The figure shows three views and two pictorial views of one solid part (mm, origin at its lowest corner). Answer the questions. Give positions to 0.01 mm unless a question says otherwise; leave off trailing zeros. Write each loop counter-clockwise with the first axis right and the second up, starting at its lowest first coordinate (ties: lowest second). Pieces come first, ordered by that corner, then holes. Notation, with made-up numbers: M 48,68 L 86,68 A28 ccw 86,107 Z; hole C 30.25,8 d10. An arc over 180 degrees is marked long. Return JSON: item names as keys, results as strings.
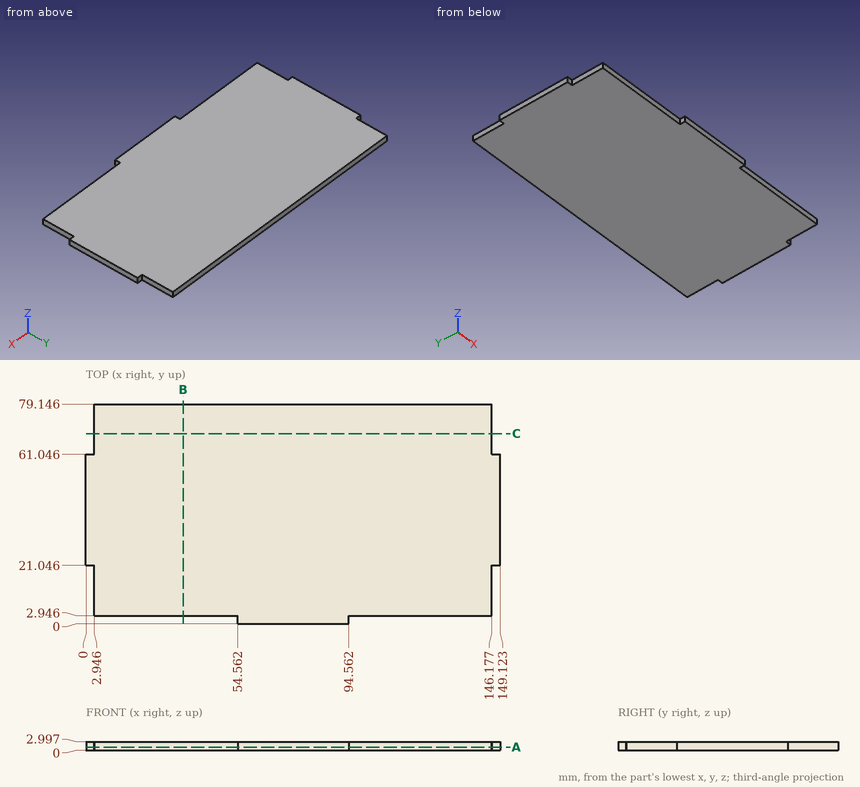
Item 1: Find the intervals of material crossed by line 1 (X direction, y = 64, z = 0.45); line 2 (Y direction, x = 96, z = 0.2), in increasing order.
Geometry results:
{"line 1": "x = 2.95 to 146.18", "line 2": "y = 2.95 to 79.15"}
Item 2: A cutting plane is placed at A-A, the plane z = 1.1. Write down the section's boundary in (x, y).
Geometry results:
{"outline": "M 0,21.05 L 2.95,21.05 L 2.95,2.95 L 54.56,2.95 L 54.56,0 L 94.56,0 L 94.56,2.95 L 146.18,2.95 L 146.18,21.05 L 149.12,21.05 L 149.12,61.05 L 146.18,61.05 L 146.18,79.15 L 2.95,79.15 L 2.95,61.05 L 0,61.05 Z"}
Item 3: Given pin 1 Ø1.5 at (x, z) = (128.5, 1.5) entering from -Y; pin 2 Ø1 at (y, z) = (20, 1.5) entering from +X; pin 3 Ø0.9 at (x, z) = (2, 1) entering from -Y, each flat-ended and moving along its own axis, determine where each tip first touches the part or whether it passes through.
Geometry results:
{"pin 1": "stops at y = 2.95", "pin 2": "stops at x = 146.18", "pin 3": "stops at y = 21.05"}
Item 4: A cutting plane is placed at C-C, the plane y = 68.5. Write down the section's boundary in (x, z).
Geometry results:
{"outline": "M 2.95,0 L 146.18,0 L 146.18,3 L 2.95,3 Z"}
Item 5: A cutting plane is placed at B-B, the plane x = 35. Write down the section's boundary in (y, z).
Geometry results:
{"outline": "M 2.95,0 L 79.15,0 L 79.15,3 L 2.95,3 Z"}
